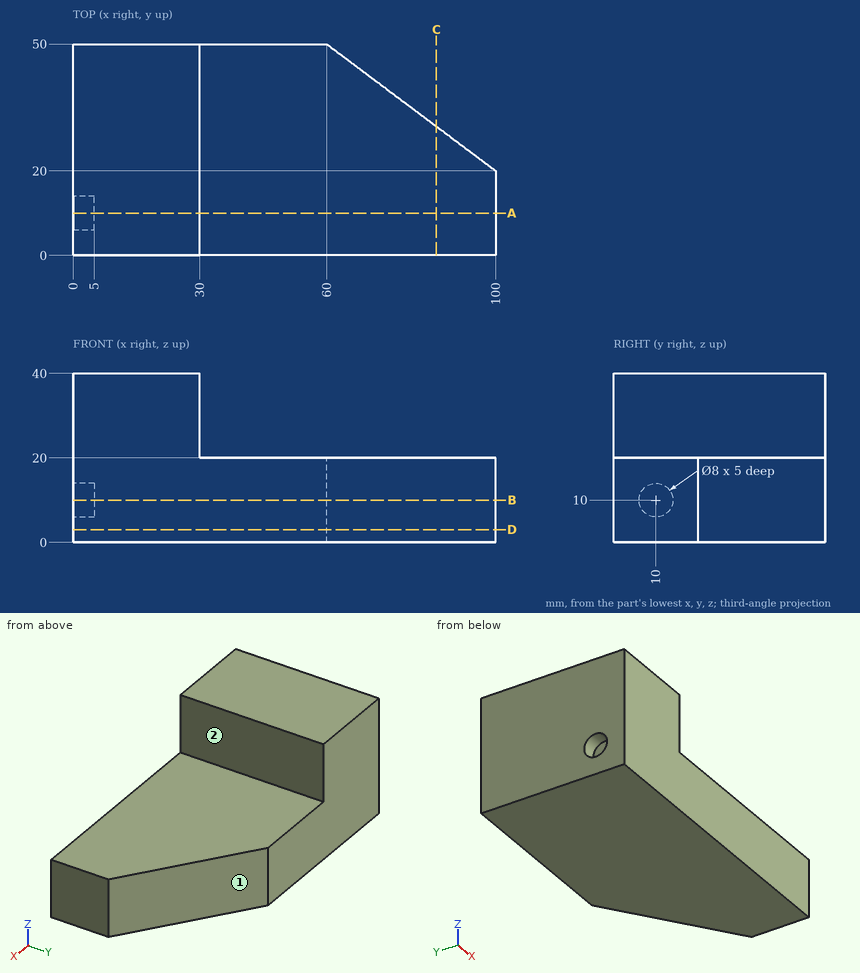
Geometry: see drawing. Coordinates: mm, zero at the bounding-box minimum. A direction names the side the tool comes from. Round coordinates to 2 decimals unless told otherwise and drop trailing zeros. Loops run counter-clockwise (first coordinate to the right, second up) from the corner with the lowest first, then second, coordinate; pieces in that order, holes last. Notation, with made-up numbers: (55.5, 78) -> (114.5, 78) arc R17 cw to (114.5, 101) -> close; hole circle Ø7 at (-33.75, 2.25). An arc over 180 degrees is marked (long way). Use one line per item in the form item = value. Start each with the question number.
Item 1: Section query C-C on x = 86. Return the cut outline in (y, z).
Item 2: Contact query for flat-ended pins moving along their axis: pin 1 Ø10 at (y, z) = (31, 29) entering from +X; pin 2 Ø25 at (x, y) = (79.5, 35) entering from +Z. Output: stop coordinate, or through.
Item 3: Section query D-D on z = 3. Return the cut outline in (x, y), then the cut area to 3 significant figures.
Item 4: Material intervals for L1, parallel to Z at x = 3, y = 10; L2, parallel to X at y = 13.5, z = 29.5; L3, parallel to Z at x = 51.5, y = 4.5, sorted ascending. Write a range as from..to.
Item 5: Section query A-A on y = 10. Return the cut outline in (x, z), then the cut area to 3 significant figures.
Item 6: Section query B-B on z = 10. Return the cut outline in (x, y).
Item 7: Set-up query: the marked faces 1 and 2. Return all of +Z, -Z, +X, -X, +Y, -Y with unobstructed straight access to the full face (end or side cutting, diameter ignored); none if empty.
Ans:
q1.outline = (0, 0) -> (30.5, 0) -> (30.5, 20) -> (0, 20) -> close
q2.pin_1 = 30
q2.pin_2 = 20
q3.outline = (0, 0) -> (100, 0) -> (100, 20) -> (60, 50) -> (0, 50) -> close
q3.area = 4,400 mm^2
q4.L1 = 0..6, 14..40
q4.L2 = 0..30
q4.L3 = 0..20
q5.outline = (0, 0) -> (100, 0) -> (100, 20) -> (30, 20) -> (30, 40) -> (0, 40) -> (0, 14) -> (5, 14) -> (5, 6) -> (0, 6) -> close
q5.area = 2,560 mm^2
q6.outline = (0, 0) -> (100, 0) -> (100, 20) -> (60, 50) -> (0, 50) -> (0, 14) -> (5, 14) -> (5, 6) -> (0, 6) -> close
q7.face_1 = +Z, -Z, +X, +Y
q7.face_2 = +Z, +X, +Y, -Y
